Input: part model. Units: mm. Frame: model coordinates. Face numbers are marked on the shaded views. A direction names the side the tool comes from. Coordinates: 2 decimals unless noted, no trailing zeros. Loops run counter-clockwise (first coordinate to the right, second up) from the corner with the lowest first, then second, coordinate; pieces in that order, holes last.
(1) Set-up query: the marked faces 5, 6 and 7. Return all of +Z, -Z, +X, -X, +Y, -Y with unobstructed straight access to the full face (end or side cutting, diameter ignored); none if empty.
(2) Section A-A, the plane z = 47. Return loops of the section in (x, y).
(3) Section D-D, the plane x = -21.5. Return loops of the section in (y, z), then the cut area to 3 significant figures.
(4) Contact query for flat-ended pins moving along their axis: P1, Ø14, axis at y = -24, z = 23, coming from the +X side; P2, Ø1.5, axis at x = -29.5, y = -45, coming from the +Z side; P3, Ø5, axis at x = -36.5, y = -60.5, coming from the +Z side; P4, Ø6.5, axis at x = -18.5, y = -65.5, coming from the +Z side. Output: stop coordinate, or through.
(5) Section C-C, the plane y = -16. Return loops of the section in (x, z), then the cut area to 3 significant figures.
(6) Line query: L1, parallel to X at y = -55.5, z = 36; L2, parallel to X at y = -73, z = 15; L3, parallel to Z at x = 14.5, y = -30. Output: solid intervals per line, ascending.
(7) Section B-B, the plane z = 31.5. Return loops of the section in (x, y).
(8) Mould query, pull axis X, two halves, no side actions, for the marked faces 1, 2, 3 and 4. Classes: released by +X, released by -X, zero draft, split by the parting line, or undercut.
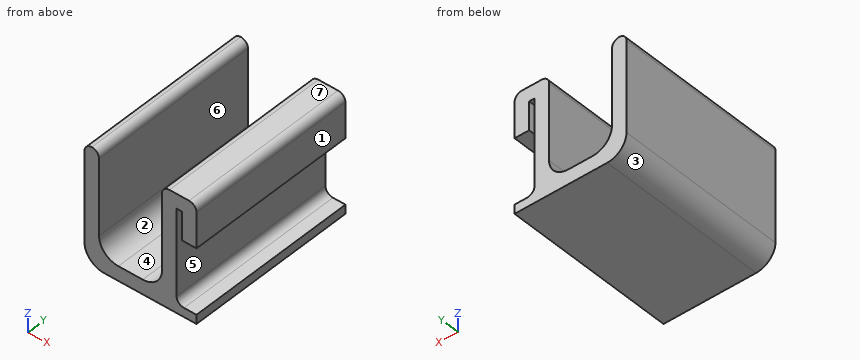
```python
from build123d import *

# Parameters (mm, degrees)
F1_DEPTH    = 95
F2_T1_DEPTH = 95
F2_T3_DEPTH = 115.5208152802
F3_R        = 10.6225396744


# Not quite as in the source:
# - a fillet or chamfer that OpenCascade refuses, or shapes differently, is made with other operations: its cross-section is extruded or revolved along the edge and cut away or added


with BuildPart() as f1:
    # F0 (on Front) → F1 (new body)
    with BuildSketch(Plane.XZ):
        Polygon((0, 56.5581262502), (0, 0), (-34.6262017979, 0), (-34.6262017979, 56.5581262502), (-42.6262017979, 56.5581262502), (-42.6262017979, -8), (8, -8), (19, -8), (19, -3), (8, -3), (8, 48.5581262502), (11, 48.5581262502), (11, 32.9302263872), (19.0000018427, 32.9302263872), (19.0000018427, 56.5581262502), align=None)
    extrude(amount=F1_DEPTH)

    # F2: fillet of radius 4.104163056 on 5 edges, made by hand

    # F2_s2 → F2_t1 (join)
    with BuildSketch(Plane.XZ):
        with BuildLine():
            ThreePointArc((8, 1.104163056), (9.202081528, -1.797918472), (12.104163056, -3))
            Line((12.104163056, -3), (8, -3))
            Line((8, -3), (8, 1.104163056))
        make_face()
    extrude(amount=F2_T1_DEPTH)

    # F2_s4 → F2_t3 (cut)
    with BuildSketch(Plane.XZ.offset(-10.2604076401)):
        with BuildLine():
            ThreePointArc((-38.5220387419, 56.5581262502), (-41.4241202699, 55.3560447222), (-42.6262017979, 52.4539631941))
            Line((-42.6262017979, 52.4539631941), (-42.6262017979, 56.5581262502))
            Line((-42.6262017979, 56.5581262502), (-38.5220387419, 56.5581262502))
        make_face()
        with BuildLine():
            ThreePointArc((-34.6262017979, 52.4539631941), (-35.828283326, 55.3560447222), (-38.730364854, 56.5581262502))
            Line((-38.730364854, 56.5581262502), (-34.6262017979, 56.5581262502))
            Line((-34.6262017979, 56.5581262502), (-34.6262017979, 52.4539631941))
        make_face()
        with BuildLine():
            ThreePointArc((0, 52.4539631941), (1.202081528, 55.3560447222), (4.104163056, 56.5581262502))
            Line((4.104163056, 56.5581262502), (0, 56.5581262502))
            Line((0, 56.5581262502), (0, 52.4539631941))
        make_face()
        with BuildLine():
            ThreePointArc((14.8958387867, 56.5581262502), (17.7979203147, 55.3560447222), (19.0000018427, 52.4539631941))
            Line((19.0000018427, 52.4539631941), (19.0000018427, 56.5581262502))
            Line((19.0000018427, 56.5581262502), (14.8958387867, 56.5581262502))
        make_face()
    extrude(amount=F2_T3_DEPTH, mode=Mode.SUBTRACT)

    # F3
    f3_edges = [f1.edges().sort_by_distance(p)[0] for p in [
        (-34.626202, -47.5, 0),
        (0, -47.5, 0),
        (-42.626202, -47.5, -8),
    ]]
    fillet(f3_edges, radius=F3_R)


solid = f1.part
```
Report:
1. face 5: +Y, -Y
1. face 6: +Z, +Y, -Y
1. face 7: +Z, +X, -X, +Y, -Y
2. outline: (-42.63, -95) - (-34.63, -95) - (-34.63, 0) - (-42.63, 0) - close; (0, -95) - (8, -95) - (8, 0) - (0, 0) - close; (11, -95) - (19, -95) - (19, 0) - (11, 0) - close
3. outline: (-95, -8) - (0, -8) - (0, 0) - (-95, 0) - close
3. area: 760 mm2
4. P1: stops at x = 8
4. P2: stops at z = 2.03
4. P3: stops at z = 56.56
4. P4: stops at z = 0
5. outline: (-42.63, 2.62) arc R10.62 ccw to (-32, -8) - (19, -8) - (19, -3) - (12.1, -3) arc R4.1 cw to (8, 1.1) - (8, 48.56) - (11, 48.56) - (11, 32.93) - (19, 32.93) - (19, 52.45) arc R4.1 ccw to (14.9, 56.56) - (4.1, 56.56) arc R4.1 ccw to (0, 52.45) - (0, 10.62) arc R10.62 cw to (-10.62, 0) - (-24, 0) arc R10.62 cw to (-34.63, 10.62) - (-34.63, 52.45) arc R4.1 ccw to (-38.63, 56.56) arc R4.1 ccw to (-42.63, 52.45) - close
5. area: 1,590 mm2
6. L1: x = -42.63 to -34.63, 0 to 8, 11 to 19
6. L2: x = -42.63 to -34.63, 0 to 8
6. L3: z = -8 to -3, 32.93 to 56.56
7. outline: (-42.63, -95) - (-34.63, -95) - (-34.63, 0) - (-42.63, 0) - close; (0, -95) - (8, -95) - (8, 0) - (0, 0) - close
8. face 1: released by +X
8. face 2: undercut
8. face 3: released by -X
8. face 4: undercut
